Verification items for this drawing (mm, ordinates from the low corner). A direction names the side the tool comes from. Round coordinates to 2 decimals unless told otherwise and drop trailing zeros. Write each loop counter-clockwise with the first axis right and the second up, starting at its lowest first coordinate (ties: lowest second). Pieces come first, ordered by that corner, then holes. Notation, with made-up numbers: M 61.5,-0.75 L 85.5,-0.75 A22 cw 85.5,32.25 Z; hole C 88,-23 d6. An arc over 180 degrees is marked long. Write each question's results on one line, items separated by ' | '.
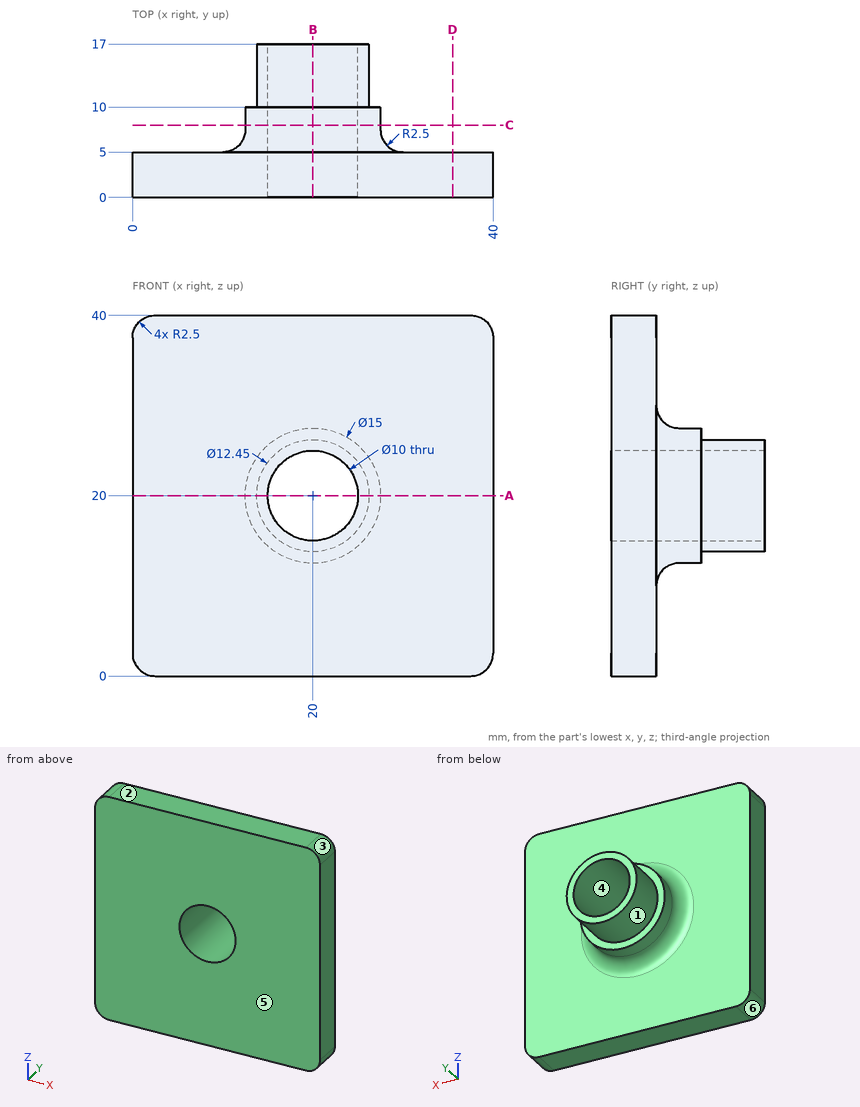
1) Draft check along X on the marked faces 3, 4, 5 and 6. Enter one of: pulls with the +X half, pulls with the -X half, needs draft (parallel to the pull), parting line crosses it, or undercut.
Calculated:
face 3: pulls with the +X half | face 4: undercut | face 5: needs draft | face 6: pulls with the -X half
2) Sectioned sample at A-A, the plane z = 20. Record the cut outline in (x, y) (3 decimals), and give its area (3 significant figures).
Calculated:
outline: M 0,0 L 15,0 L 15,17 L 13.775,17 L 13.775,10 L 12.5,10 L 12.5,7.5 A2.5 cw 10,5 L 0,5 Z; M 25,0 L 40,0 L 40,5 L 30,5 A2.5 cw 27.5,7.5 L 27.5,10 L 26.225,10 L 26.225,17 L 25,17 Z | area: 195 mm²
3) Sectioned sample at D-D, the plane x = 35.5. Record the cut outline in (y, z).
Calculated:
outline: M 0,0 L 5,0 L 5,40 L 0,40 Z
4) Sectioned sample at C-C, the plane y = 8. Record the cut outline in (x, z), and give its area (3 significant figures).
Calculated:
outline: C 20,20 d15; hole C 20,20 d10 | area: 98.2 mm²
5) Material ranges on line 1 (X direction, y = 11.25, z = 20) (3 decimals); line 2 (Y direction, x = 5, z = 38); line 3 (Z direction, x = 23, y = 10.5), recorded low to high. Write a range as [from, to].
Calculated:
line 1: x = [13.775, 15], [25, 26.225] | line 2: y = [0, 5] | line 3: z = [14.55, 16], [24, 25.45]
6) Depth check by flat-ended pin: P1, Ø6, axis at y = 13.5, z = 27, coming from the +X side; P2, Ø3, axis at x = 26.5, z = 14, coming from the +Y side; P3, Ø3, axis at x = 17, y = 7.5, coming from the +Z side. Enter the tip coordinate at first touch or a pass-through.
Calculated:
P1: stops at x = 24.77 | P2: stops at y = 10 | P3: stops at z = 27.54
7) Sectioned sample at B-B, the plane x = 20. Record the cut outline in (y, z) (3 decimals).
Calculated:
outline: M 0,0 L 5,0 L 5,10 A2.5 cw 7.5,12.5 L 10,12.5 L 10,13.775 L 17,13.775 L 17,15 L 0,15 Z; M 0,25 L 17,25 L 17,26.225 L 10,26.225 L 10,27.5 L 7.5,27.5 A2.5 cw 5,30 L 5,40 L 0,40 Z
8) Access from +Z, -Z, +X, -X, +Y, -Y to the whole of each face (thin tool, end or side, straight path). Record for the marked faces 1 and 2.
Calculated:
face 1: +Y | face 2: +Z, +X, -X, +Y, -Y
